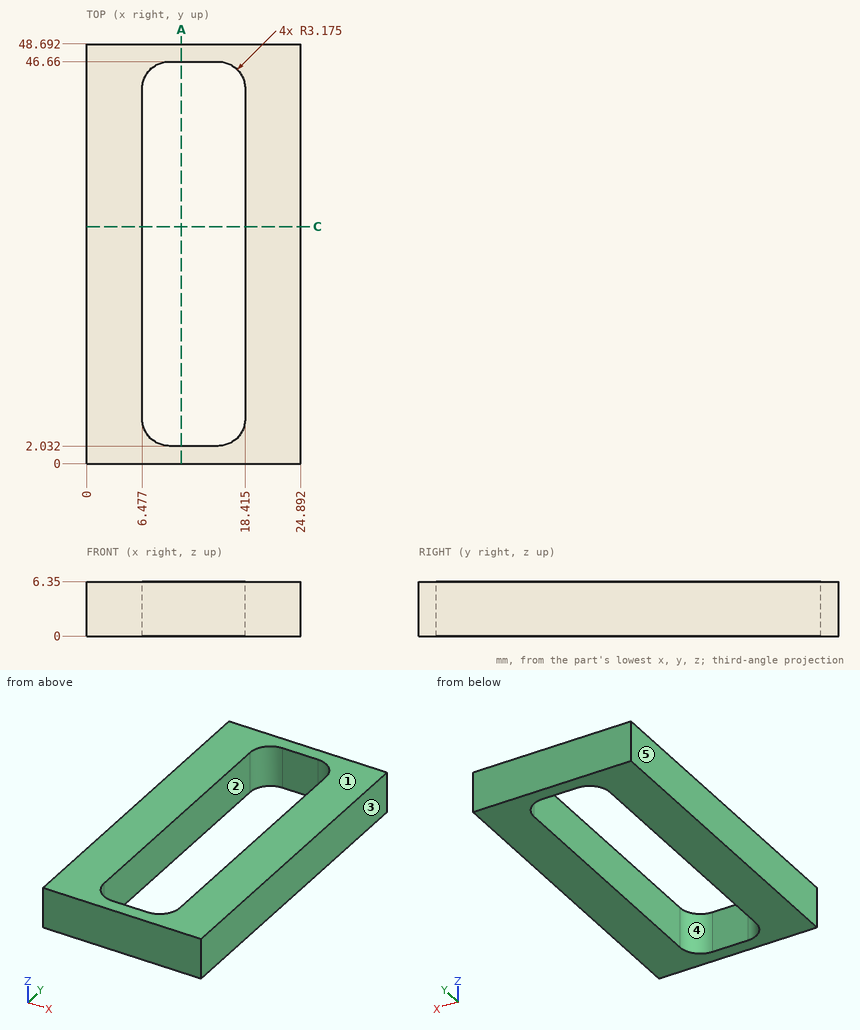
Print and shaded views of the part. All mm, measured from the part's lowest x, y and z. A direction names the side the tool comes from. Coordinates: 2 decimals unless noted, no trailing zeros. Loops run counter-clockwise (first coordinate to the right, second up) from the corner with the lowest first, then second, coordinate; pieces in that order, holes last. Notation, with made-up numbers: (60.25, 61.25) -> (109.25, 61.25) arc R17 ccw to (109.25, 85.25) -> close; hole circle Ø6 at (67, -35.75). An arc over 180 degrees is marked (long way). Use one line per item in the form item = value. Start each with the question number.
(1) Probe probe 1 along X at (y, z) = (35, 1.75) (3 decimals); probe 2 along Y at (x, z) = (15.25, 2.75); probe 3 along Y at (x, z) = (17.5, 2) (1 decimal). List the from-to ranges inside material, lowest first. Write a range as from..to.
(2) Tool access for the marked faces 4 and 5: list every direction of +Z, -Z, +X, -X, +Y, -Y with a clear straight run to the whole face (end or side of a thin tool).
(3) Cut at A-A on x = 11. Give the cut face in (y, z), and give its area (3 significant figures).
(4) Cut at C-C on y = 27.5. Give the cut face in (x, z) (3 decimals).
(5) Flat gauge pin, fed straight in: pin 1 (3 mm diameter, centred on y = 20, z = 4.5, fed in from -X). Where does the tip first touch, or does it go through?
(6) Pull direction X, two halves, no side cores. Call the marked faces 1, 2 and 3: pulls with the +X half, pulls with the -X half, needs draft (parallel to the pull), parting line crosses it, or undercut.
Values:
q1.probe_1 = 0..6.477, 18.415..24.892
q1.probe_2 = 0..2.03, 46.66..48.69
q1.probe_3 = 0..3, 45.7..48.7
q2.face_4 = +Z, -Z
q2.face_5 = +Z, -Z, -X, +Y, -Y
q3.outline = (0, 0) -> (2.03, 0) -> (2.03, 6.35) -> (0, 6.35) -> close; (46.66, 0) -> (48.69, 0) -> (48.69, 6.35) -> (46.66, 6.35) -> close
q3.area = 25.8 mm2
q4.outline = (0, 0) -> (6.477, 0) -> (6.477, 6.35) -> (0, 6.35) -> close; (18.415, 0) -> (24.892, 0) -> (24.892, 6.35) -> (18.415, 6.35) -> close
q5.pin_1 = 0
q6.face_1 = needs draft
q6.face_2 = undercut
q6.face_3 = pulls with the +X half
